Here's how the part is built. I have some questions about the finished solid (model axes, mm). Coordinates: 2 decimals unless noted, no trailing zeros. Write each loop counter-clockwise with the first axis right and the second up, starting at its lowest first coordinate (ties: lowest second). Pieces come first, ordered by that corner, then holes. Notation, with made-up numbers: M -33,79.5 L 13,79.5 A9 ccw 13,95.5 Z; hole C 0.5,-31 d7. An arc over 180 degrees is marked long. Write each question's results on one line, items separated by ' | '. Start each with the question number.
Autodesk Inventor part; units mm, degrees
ref_plane "YZ Plane" through (0, 0, 0) normal (1, 0, 0) x (0, 1, 0)
ref_plane "XZ Plane" through (0, 0, 0) normal (0, 1, 0) x (-1, 0, 0)
ref_plane "XY Plane" through (0, 0, 0) normal (0, 0, 1) x (1, 0, 0)
sketch "Sketch1" plane through (0, 0, 0) normal (0, 1, 0) x (-1, 0, 0)
  line L0 (7.3323, 0) -> (3.6662, -6.35)
  line L1 (3.6662, -6.35) -> (-3.6662, -6.35)
  line L2 (-3.6662, -6.35) -> (-7.3323, 0)
  line L3 (-7.3323, 0) -> (-3.6662, 6.35)
  line L4 (-3.6662, 6.35) -> (3.6662, 6.35)
  line L5 (3.6662, 6.35) -> (7.3323, 0)
  circle A0 centre (0, 0) radius 2.5527
  circle A1 centre (0, 0) radius 6.8758
  point P0 (2.637, -6.35)
  point P1 (4.1808, -5.4587)
  point P2 (6.8178, -0.8913)
  point P3 (6.8178, 0.8913)
  point P4 (4.1808, 5.4587)
  point P5 (2.637, 6.35)
  point P6 (-2.637, 6.35)
  point P7 (-4.1808, 5.4587)
  point P8 (-6.8178, 0.8913)
  point P9 (-6.8178, -0.8913)
  point P10 (-4.1808, -5.4587)
  point P11 (-2.637, -6.35)
  dimension "d0" = 6.35
  dimension "d1" = 5.1054
  dimension "d2" = 13.7516
extrude "Extrusion1" add sketch "Sketch1" along normal blind 914.4 contours L0 A1 L1 L2 L3 L4 L5
properties part number "thunder hex 36in"
1) I want a section at A-A, the plane x = 0. Write out the boundary of the cut face in (y, z).
2) Please list where these lines run through material, in increasing order: line 1 (Z direction, x = 0, y = 394.5); line 2 (Z direction, x = 0.75, y = 740); line 3 (X direction, y = 117.5, z = -0.75). Write a range as [from, to].
3) I want a section at B-B, the plane y = 132. Write out the boundary of the cut face in (x, z), then the cut area to 3 significant figures.
4) For pin 1 Ø3 at (y, z) = (105.5, -3.5) entering from +X; pin 2 Ø1.5 at (y, z) = (105.5, -3) entering from +X; pin 3 Ø4.5 at (x, z) = (0, 0) entering from -Y, each with a flat end and sliding along its axis, tell me the tip position at first contact or that it passes through.
Output:
1) outline: M 0,-6.35 L 914.4,-6.35 L 914.4,-2.55 L 0,-2.55 Z; M 0,2.55 L 914.4,2.55 L 914.4,6.35 L 0,6.35 Z
2) line 1: z = [-6.35, -2.55], [2.55, 6.35] | line 2: z = [-6.35, -2.44], [2.44, 6.35] | line 3: x = [-6.83, -2.44], [2.44, 6.83]
3) outline: M -6.82,-0.89 L -4.18,-5.46 A6.88 ccw -2.64,-6.35 L 2.64,-6.35 A6.88 ccw 4.18,-5.46 L 6.82,-0.89 A6.88 ccw 6.82,0.89 L 4.18,5.46 A6.88 ccw 2.64,6.35 L -2.64,6.35 A6.88 ccw -4.18,5.46 L -6.82,0.89 A6.88 ccw Z; hole C 0,0 d5.11 | area: 117 mm2
4) pin 1: stops at x = 6.18 | pin 2: stops at x = 6.03 | pin 3: passes through
